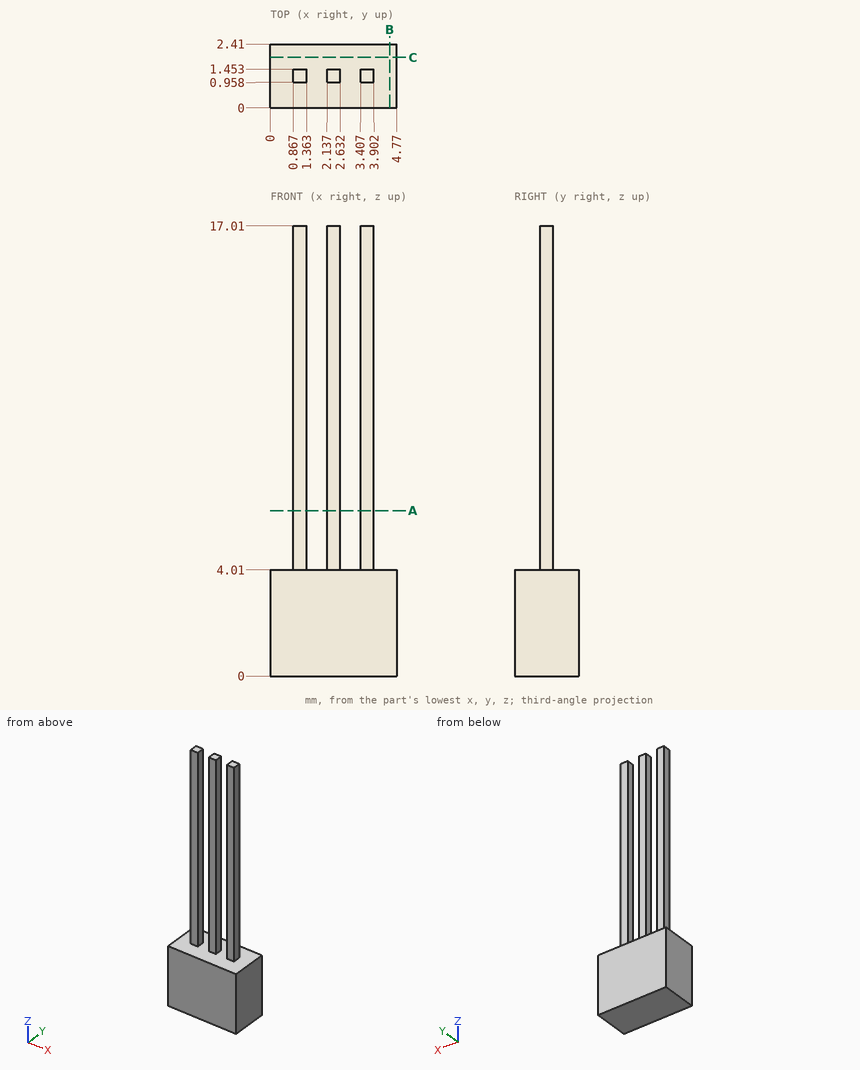
Drawing for the job (mm, zero at the part's lowest x, y, z). Give positions to 0.01 mm unless a question says otherwise; leave off trailing zeros. Order: outer loops, then holes, each group sorted by start corner. A loop starts at its lowest first (then second) coordinate and runs counter-clockwise, first axis right, second up. Notation, with made-up numbers: (60, -38) - (69, -38) arc R24 cw to (69, -16) - close; hole circle Ø9 at (13, 66.5). An arc over 180 degrees is marked (long way). Write item = value, one per line. Start each with the question number.
1. Cut at C-C, the plane y = 1.9. List the corners of the cut face in (x, z).
2. Cut at B-B, the plane x = 4.5. List the corners of the cut face in (y, z).
3. Probe line 1 along X through (y, z) = (1.15, 5.75); line 2 along Y through (x, z) = (2.4, 13.25); line 3 along Z through (x, y) = (0.5, 1.5). List the from-to ranges inside material, lowest first.
4. Cut at A-A, the plane z = 6.25. List the corners of the cut face in (x, y).
5. Drop flat-ended pins along their axis: P1, Ø0.5, axis at x = 2.5, z = 9, coming from the +Y side; P2, Ø0.5, axis at y = 1.5, z = 12, coming from the +X side; P3, Ø0.5, axis at x = 4, z = 7.5, coming from the -Y side. Give the stop position or say it passes through.
Taken from the geometry:
q1.outline = (0, 0) - (4.77, 0) - (4.77, 4.01) - (0, 4.01) - close
q2.outline = (0, 0) - (2.41, 0) - (2.41, 4.01) - (0, 4.01) - close
q3.line_1 = 0.87 to 1.36, 2.14 to 2.63, 3.41 to 3.9
q3.line_2 = 0.96 to 1.45
q3.line_3 = 0 to 4.01
q4.outline = (0.87, 0.96) - (1.36, 0.96) - (1.36, 1.45) - (0.87, 1.45) - close; (2.14, 0.96) - (2.63, 0.96) - (2.63, 1.45) - (2.14, 1.45) - close; (3.41, 0.96) - (3.9, 0.96) - (3.9, 1.45) - (3.41, 1.45) - close
q5.P1 = 1.45
q5.P2 = 3.9
q5.P3 = 0.96
